Here's the drawing with two shaded views (mm, measured from the low corner). I have some questions. A direction names the side the tool comes from. Coordinates: 2 decimals unless noted, no trailing zeros. Write each loop counter-clockwise with the first axis right and the second up, starting at its lowest first coordinate (ties: lowest second). Pieces come first, ordered by that corner, then holes. Notation, with made-up numbers: (6.5, -10) - (62.5, -10) arc R19 cw to (62.5, 16) - close; hole circle Ø9 at (-20.75, 73). An arc over 180 degrees is marked (long way). Answer in a Markdown table with one row per item. Add a question column.
Item 1: If I drill on probe 1 along X at (y, z) = (5.25, 1); probe 2 along Y at (x, z) = (23.5, 3.75), over which ranges is the centre line in solid material (lowest first)? Write a range as from..to.
Item 2: Imagine slicing it at A-A (x = 16). Please give me the cut outline in (y, z).
Item 3: I'm going to push flat-ended pins straight in: pin 1 (1 mm diameter, centred on x = 5, y = 4, fed in from -Z); pin 2 (1.5 mm diameter, centred on x = 20, y = 1, fed in from -Z); pin 3 (1.9 mm diameter, centred on y = 2.5, z = 3.5, fed in from -X); pin 4 (3 mm diameter, centred on x = 24, y = 1, fed in from +Z). Where does each tip first touch, or does it pass through?
Item 4: Which directions (+Z, -Z, +X, -X, +Y, -Y) give clear straight access to the entire face, cutting with the end or side of a thin tool? Please do the marked faces 1 and 2.
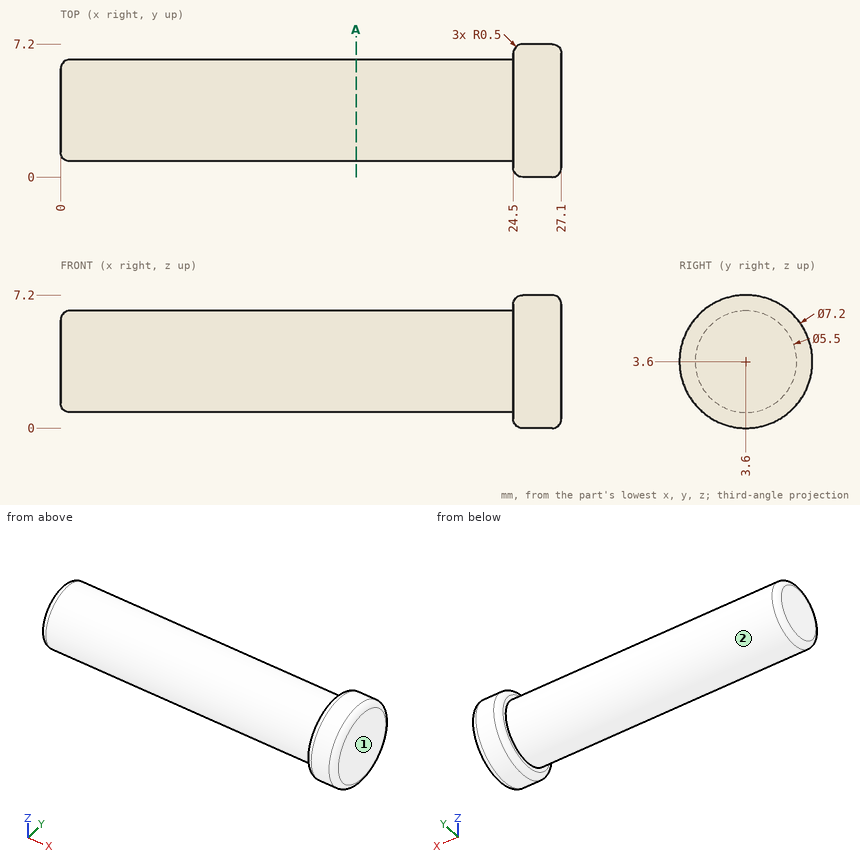
Here are the results:
| question | item | result |
|---|---|---|
| 1 | probe 1 | x = 24.5..27.1 |
| 1 | probe 2 | y = 0.85..6.35 |
| 2 | outline | circle Ø5.5 at (3.6, 3.6) |
| 3 | pin 1 | stops at z = 0.85 |
| 3 | pin 2 | stops at z = 1.57 |
| 3 | pin 3 | stops at x = 0 |
| 3 | pin 4 | stops at z = 6.91 |
| 4 | face 1 | +Z, -Z, +X, +Y, -Y |
| 4 | face 2 | -X |
